Autodesk Fusion 360 part; units mm, degrees
sketch "Sketch1" plane through (0, 0, 0) normal (0, 0, 1) x (1, 0, 0)
  line L0 (0, 0) -> (44.95, 0)
  line L1 (44.95, 0) -> (44.95, 14.95)
  line L2 (44.95, 14.95) -> (0, 14.95)
  line L3 (0, 14.95) -> (0, 0)
  line L4 (5, 5) -> (39.95, 5)
  line L5 (39.95, 5) -> (39.95, 9.95)
  line L6 (39.95, 9.95) -> (5, 9.95)
  line L7 (5, 9.95) -> (5, 5)
  dimension "d1" = 44.95
  dimension "d2" = 14.95
  dimension "d3" = 34.95
  dimension "d4" = 4.95
  dimension "d5" = 5
  dimension "d6" = 5
extrude "Extrude1" add sketch "Sketch1" along normal blind 12 contours L4 L5 L6 L7
extrude "Extrude2" add sketch "Sketch1" along normal blind 2
sketch "Sketch2" plane through (0, 0, 2) normal (0, 0, 1) x (-1, 0, 0)
  line L0 (-5, -5) -> (-5, -9.95)
  line L1 (-5, -9.95) -> (-39.95, -9.95)
  line L2 (-39.95, -9.95) -> (-39.95, -5)
  line L3 (-39.95, -5) -> (-5, -5)
  line L4 (0, -14.95) -> (0, 0)
  line L5 (0, 0) -> (-44.95, 0)
  line L6 (-44.95, 0) -> (-44.95, -14.95)
  line L7 (-44.95, -14.95) -> (0, -14.95)
  line L8 (-44.95, 0) -> (0, 0)
  line L9 (0, 0) -> (0, -5)
  line L10 (0, -5) -> (-44.95, -5)
  line L11 (-44.95, -5) -> (-44.95, 0)
extrude "Extrude3" cut sketch "Sketch2" against normal blind 4 contours L3 L4 L5 L6 L8 L9 L10 L11
Could you check a few things on this model? Use its own coordinates, in mm. A direction names the side the tool comes from. Coordinates: 2 decimals unless noted, no trailing zeros. Order: outer loops, then holes, each group sorted by start corner. A loop starts at its lowest first (then second) coordinate and runs counter-clockwise, first axis right, second up.
Q1. Suppose I cut it at D-D on y = 12. Please give me the cut outline in (x, z).
Q2. Suppose I cut it at B-B on x = 22. Please give me the cut outline in (y, z).
Q3. Which directions (+Z, -Z, +X, -X, +Y, -Y) give clear straight access to the entire face, cutting with the end or side of a thin tool? Please do faces 1 (the flat face through (39.95, 7, 7)), 2 (the flat face through (5, 8, 7)), 3 (the flat face through (23, 9.95, 7)).
Q4. Will these pins go through, and if not, where does the flat tip stop? pin 1 (3 mm diameter, centred on x = 25.5, z = 7, fed in from +Y); pin 2 (5 mm diameter, centred on x = 24.5, y = 10, fed in from +Z); pin 3 (5.5 mm diameter, centred on y = 7, z = 7.5, fed in from -X); pin 4 (5.5 mm diameter, centred on y = 8.5, z = 6, fed in from +X).
Q5. Suppose I cut it at A-A on y = 7. Please give me the cut outline in (x, z), and give its area (3 significant figures).
Q6. Please list where these lines run through material, in increasing order: L1, parallel to X at y = 6.25, z = 7.25; L2, parallel to Y at x = 33, z = 8; L3, parallel to Z at x = 22.5, y = 13.75.
Q7. Suppose I cut it at C-C on z = 6.75. Please give me the cut outline in (x, y).
Answer:
1. outline: (0, 0) - (44.95, 0) - (44.95, 2) - (0, 2) - close
2. outline: (5, 0) - (14.95, 0) - (14.95, 2) - (9.95, 2) - (9.95, 12) - (5, 12) - close
3. face 1: +Z, +X, +Y, -Y
3. face 2: +Z, -X, +Y, -Y
3. face 3: +Z, +X, -X, +Y
4. pin 1: stops at y = 9.95
4. pin 2: stops at z = 12
4. pin 3: stops at x = 5
4. pin 4: stops at x = 39.95
5. outline: (0, 0) - (44.95, 0) - (44.95, 2) - (39.95, 2) - (39.95, 12) - (5, 12) - (5, 2) - (0, 2) - close
5. area: 439 mm2
6. L1: x = 5 to 39.95
6. L2: y = 5 to 9.95
6. L3: z = 0 to 2
7. outline: (5, 5) - (39.95, 5) - (39.95, 9.95) - (5, 9.95) - close
